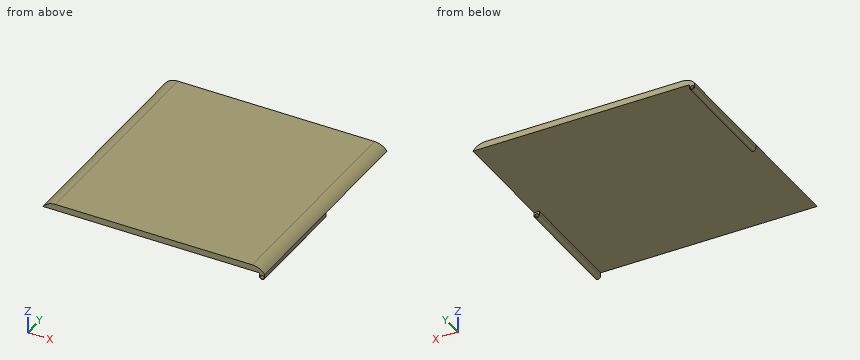
from build123d import *

# Parameters (mm, degrees)
F1_W     = 914.4
F1_H     = 914.4
F2_DEPTH = 25.4
F4_DEPTH = 914.4
F6_R     = 7.62
F7_DEPTH = 457.2
F8_DEPTH = 457.2


with BuildPart() as f2:
    # F1 (on offset) → F2 (new body)
    with BuildSketch(Plane.XY.offset(914.4)):
        Rectangle(F1_W, F1_H)
    extrude(amount=-F2_DEPTH)

    # F3 (on face) → F4 (cut, through all)
    with BuildSketch(Plane.XZ.offset(457.2)):
        with BuildLine():
            ThreePointArc((-457.2, 889), (-434.4934859844, 907.702903129), (-405.8485342879, 914.4))
            Line((-405.8485342879, 914.4), (-457.2, 914.4))
            Line((-457.2, 914.4), (-457.2, 889))
        make_face()
        with BuildLine():
            Line((457.2, 889), (457.2, 914.4))
            Line((457.2, 914.4), (405.8485342879, 914.4))
            ThreePointArc((405.8485342879, 914.4), (434.4934859844, 907.702903129), (457.2, 889))
        make_face()
    extrude(amount=-F4_DEPTH, mode=Mode.SUBTRACT)

    # F6 (on Front) → F7 (join, through all)
    with BuildSketch(Plane.XZ):
        with BuildLine():
            Line((-457.2, 889), (-457.2, 874.268))
            ThreePointArc((-457.2, 874.268), (-446.532, 863.6), (-435.864, 874.268))
            Line((-435.864, 874.268), (-435.864, 889))
            Line((-435.864, 889), (-457.2, 889))
        make_face()
        with Locations((-446.532, 874.268)):
            Circle(F6_R, mode=Mode.SUBTRACT)
    extrude(amount=-F7_DEPTH)

    # F6 (on Front) → F8 (join, through all)
    with BuildSketch(Plane.XZ):
        with BuildLine():
            Line((435.864, 889), (435.864, 874.268))
            ThreePointArc((435.864, 874.268), (446.532, 863.6), (457.2, 874.268))
            Line((457.2, 874.268), (457.2, 889))
            Line((457.2, 889), (435.864, 889))
        make_face()
        with Locations((446.532, 874.268)):
            Circle(F6_R, mode=Mode.SUBTRACT)
    extrude(amount=F8_DEPTH)


solid = f2.part
Check sheet for the modelled part. Datum: model origin and axes. Units: mm. Give positions to 0.01 mm unless a question says otherwise; leave off trailing zeros. Loops run counter-clockwise (first coordinate to the right, second up) from the corner with the lowest first, then second, coordinate; pieces in that order, holes last. Notation, with made-up numbers: M 26.5,41.5 L 50.5,41.5 A25 cw 50.5,66.5 Z; hole C 43.5,6 d3. An arc over 180 degrees is marked long. Use a Markdown table: item, result. Add a question column.
Q1. Sectioned sample at A-A, the plane y = -222.5. Record the cut outline in (x, z), then the cut area to 3 significant figures.
Q2. Scan lines: line 1 along Z through (x, y) = (-269.5, -71); line 2 along X through (y, z) = (102, 887); line 3 along X through (y, z) = (288.5, 907). Record each from-to range of solid material in increasing order. Write a range as [from, to].
Q3. Go/stop test with flat-tipped pins: pin 1 (1 mm diameter, centred on y = -264, z = 879.5, fed in from -X); pin 2 (17.5 mm diameter, centred on x = -446.532, z = 874.268, fed in from -Y); pin 3 (1.5 mm diameter, centred on y = -198.5, z = 891, fed in from -X). Record where each tip stops, or that it passes through.
Q4. Sectioned sample at B-B, the plane x = -200. Record the cut outline in (y, z), then the cut area to 3 significant figures.
Verdict:
| question | item | result |
|---|---|---|
| 1 | outline | M -457.2,889 L 435.86,889 L 435.86,874.27 A10.67 ccw 457.2,874.27 L 457.2,889 A64.61 ccw 405.85,914.4 L -405.85,914.4 A64.61 ccw Z; hole C 446.53,874.27 d15.24 |
| 1 | area | 22,700 mm^2 |
| 2 | line 1 | [889, 914.4] |
| 2 | line 2 | [-457.2, -435.86] |
| 2 | line 3 | [-435.87, 435.87] |
| 3 | pin 1 | x = 435.86 |
| 3 | pin 2 | y = 0 |
| 3 | pin 3 | x = -456.22 |
| 4 | outline | M -457.2,889 L 457.2,889 L 457.2,914.4 L -457.2,914.4 Z |
| 4 | area | 23,200 mm^2 |
